Drawing for the job (mm, zero at the part's lowest x, y, z). A direction names the side the tool comes from. Round coordinates to 2 decimals unless told otherwise and drop trailing zeros. Write each loop counter-clockwise with the first axis right and the second up, starting at its lowest first coordinate (ties: lowest second). Pieces come first, ordered by that corner, then holes. Notation, with made-up numbers: M 29.5,16.25 L 78.5,16.25 A23 cw 78.5,45.25 Z; hole C 19.25,72 d5. An arc over 180 degrees is marked long. Use a Markdown table: item, result. Add a question column.
1) Slice it at B-B on x = 71. Write the cut outline in (y, z).
2) Drop flat-ended pins along their axis: P1, Ø5, axis at y = 12.5, z = 30, coming from the +X side; P2, Ø6, axis at y = 20.5, z = 15.5, coming from the -X side; P3, Ø5, axis at x = 76, y = 6.5, coming from the +Z side. Give the stop position or say it passes through.
3) Which spindle directions (+Z, -Z, +X, -X, +Y, -Y) get a long thin tool onto all of the face, cutting with end or side? Do the marked faces 1, 2 and 3. Say none if no direction does.
4) Wall check: probe 1 along X at (y, z) = (4.25, 12); probe 2 along X at (y, z) = (24.25, 39); probe 3 along X at (y, z) = (9.25, 30) (1 decimal). Give the ranges that are in metal, low to high.
5) Slice it at C-C on x = 40. Write the cut outline in (y, z), plus the area to 3 significant figures.
6) Slice it at A-A on y = 21.75. Write the cut outline in (x, z), plus the area to 3 significant figures.
7) Two-plate mould, pull along X, no slides. Class the marked faces 4, 5 and 6: released by +X, released by -X, zero draft, split by the parting line, or undercut.
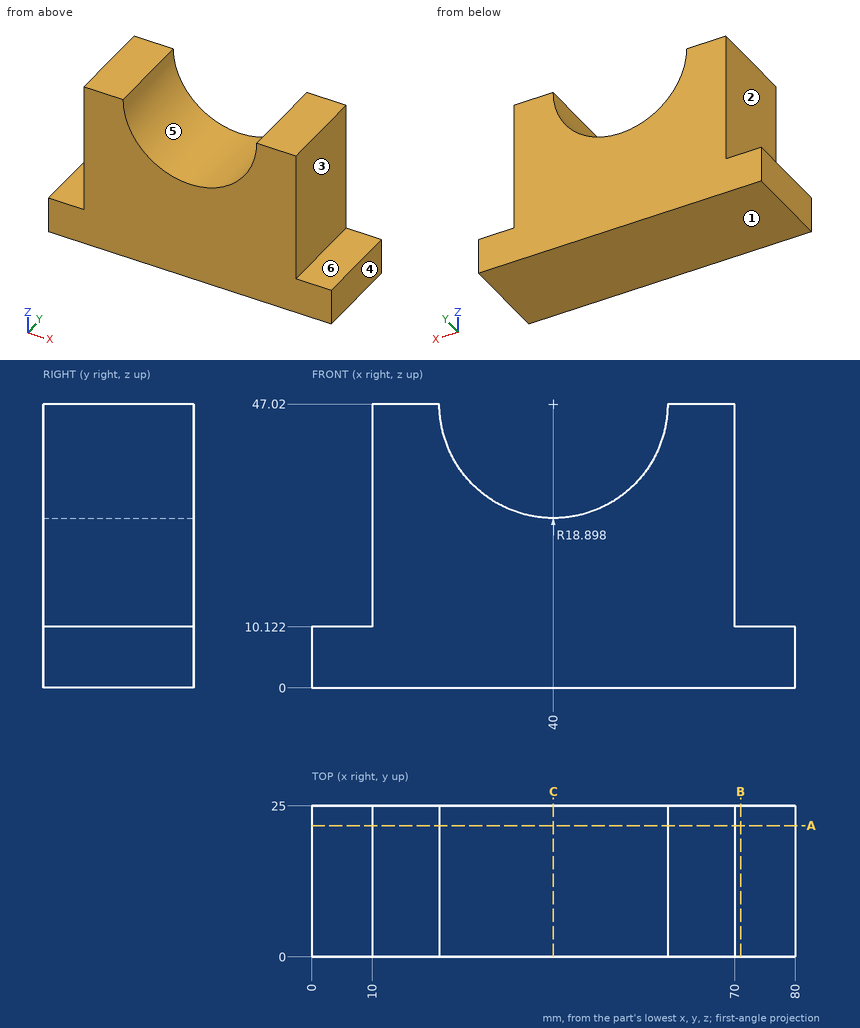
Entries:
| question | item | result |
|---|---|---|
| 1 | outline | M 0,0 L 25,0 L 25,10.12 L 0,10.12 Z |
| 2 | P1 | stops at x = 70 |
| 2 | P2 | stops at x = 10 |
| 2 | P3 | stops at z = 10.12 |
| 3 | face 1 | -Z, +X, -X, +Y, -Y |
| 3 | face 2 | +Z, -X, +Y, -Y |
| 3 | face 3 | +Z, +X, +Y, -Y |
| 4 | probe 1 | x = 10 to 70 |
| 4 | probe 2 | x = 10 to 22.89, 57.11 to 70 |
| 4 | probe 3 | x = 10 to 31.8, 48.2 to 70 |
| 5 | outline | M 0,0 L 25,0 L 25,28.12 L 0,28.12 Z |
| 5 | area | 703 mm^2 |
| 6 | outline | M 0,0 L 80,0 L 80,10.12 L 70,10.12 L 70,47.02 L 58.9,47.02 A18.9 cw 21.1,47.02 L 10,47.02 L 10,10.12 L 0,10.12 Z |
| 6 | area | 2,460 mm^2 |
| 7 | face 4 | released by +X |
| 7 | face 5 | undercut |
| 7 | face 6 | zero draft |
